Print and shaded views of the part. All mm, measured from the part's lowest x, y and z. Round coordinates to 2 decimals unless told otherwise and drop trailing zeros. Write each loop counter-clockwise with the first axis right and the second up, starting at its lowest first coordinate (ties: lowest second). Pieces come first, ordered by that corner, then holes.
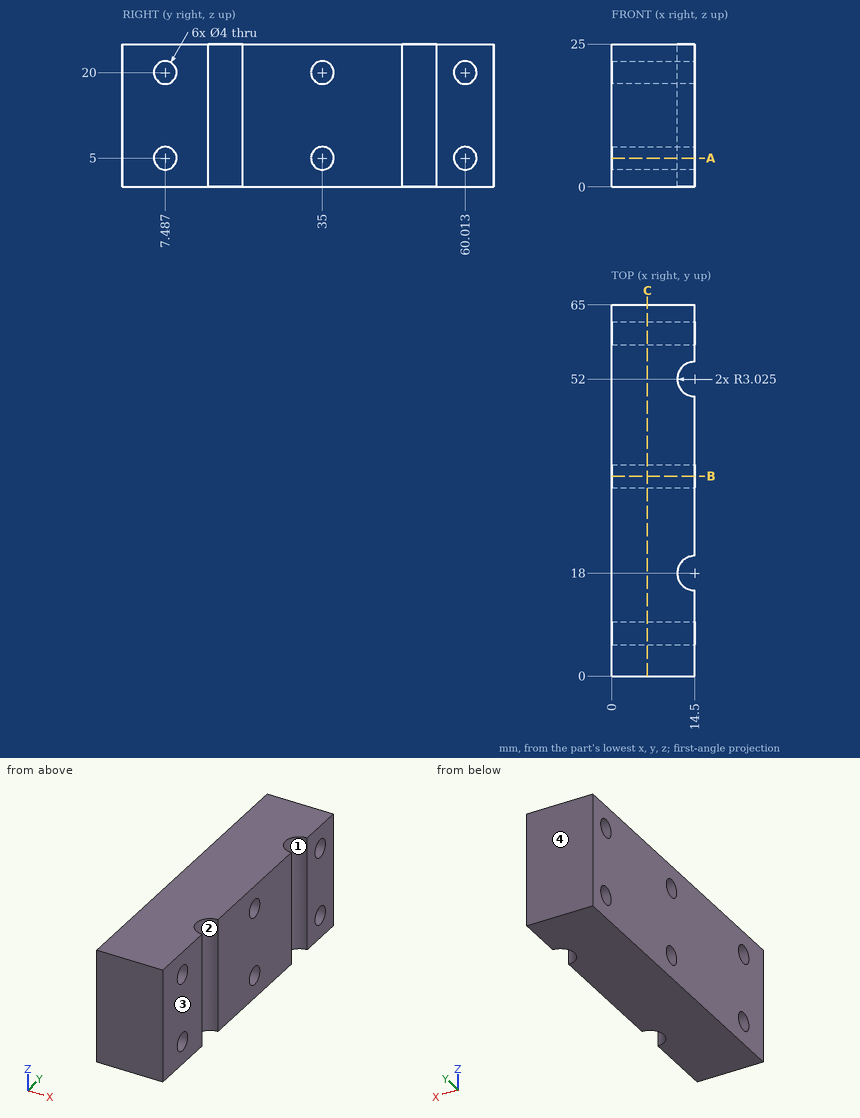
1) Slice it at A-A (z = 5). Count the separate pieces of the cut face and the enclosed holes in it, plus the area to 3 significant figures.
Results:
separate pieces: 4
enclosed holes: 0
area: 740 mm2
2) Slice it at C-C (x = 6.25). Write the cut outline in (y, z).
Results:
outline: (0, 0) - (65, 0) - (65, 25) - (0, 25) - close; hole circle Ø4 at (7.49, 5); hole circle Ø4 at (7.49, 20); hole circle Ø4 at (35, 5); hole circle Ø4 at (35, 20); hole circle Ø4 at (60.01, 5); hole circle Ø4 at (60.01, 20)
3) Mould opens along Y. For the marked faces 1, 2, 3 and 4 say: released by +Y, released by -Y, zero draft, split by the parting line, or undercut.
Results:
face 1: undercut
face 2: undercut
face 3: zero draft
face 4: released by +Y
4) Wall check: L1, parallel to Y at x = 7, z = 5; L2, parallel to Y at x = 9.75, z = 18.5 (1 decimal); L3, parallel to Y at x = 13.75, z = 8.5. Give the ranges that are in metal, low to high.
Results:
L1: y = 0 to 5.49, 9.49 to 33, 37 to 58.01, 62.01 to 65
L2: y = 0 to 6.2, 8.8 to 33.7, 36.3 to 58.7, 61.3 to 65
L3: y = 0 to 15.07, 20.93 to 49.07, 54.93 to 65
5) Slice it at B-B (y = 35). Write the cut outline in (x, z).
Results:
outline: (0, 0) - (14.5, 0) - (14.5, 3) - (0, 3) - close; (0, 7) - (14.5, 7) - (14.5, 18) - (0, 18) - close; (0, 22) - (14.5, 22) - (14.5, 25) - (0, 25) - close
